For this review, take the finished solid that the model builds, in its own axes (mm). A direction names the side the tool comes from. Coordinates: 2 decimals unless noted, no trailing zeros. Loops run counter-clockwise (first coordinate to the right, second up) from the corner with the lowest first, then second, coordinate; pieces in that order, holes last. Notation, with made-up numbers: M -20,1 L 34,1 A9 cw 34,5 Z; hole C -37,13.25 d8. An arc over 180 degrees is marked long. Answer as a JSON object with one key per item and string values. Group by question number.
Item 1: Mouldability with a two-part tool opening along X and no side actions: class faces 3 (the face through (50, 4, 0)), 4 (the face through (107.95, 38, 25)), 5 (the face through (53, 5.08, 23)) as +X half, -X half, draft (parallel to the pull), parting line (faces both ways), or undercut.
Item 2: Tool access review of faces 1 (the face through (53, 38, 45.72)), 2 (the face through (53, 76.2, 25)): name each direction out of +Z, -Z, +X, -X, +Y, -Y from which nothing blocks a thin tool from reaching the whole face with its end or side.
Item 3: Add section C-C (y = 24). State the section outline as (x, z) points.
Item 4: Add section B-B (x = 29). State the section outline as (y, z) points.
Item 5: Insertion check: pin 1 (23 mm diameter, centred on y = 40.5, z = 16.5, fed in from -X); pin 2 (4 mm diameter, centred on x = 39.5, y = 38.5, fed in from -Z). Each pin has a flat end and moves straight along its axis. Give the tip position at first contact, or say it passes through.
Item 6: Add section A-A (z = 26.5). State the section outline as (x, y) points, then the cut area to 3 significant figures.
Item 7: Wall thickness on L1, parallel to Y at x = 28, z = 16; L2, parallel to X at y = 55.5, z = 29; L3, parallel to Z at x = 57, y = 38: over which ranges is each line inside the solid? List them lowest first. Write a range as from..to.
from build123d import *

# Parameters (mm, degrees)
F0_W     = 107.95
F0_H     = 76.2
F0_W_2   = 97.79
F0_H_2   = 66.04
F1_DEPTH = 50.8
F2_W     = 97.79
F2_H     = 66.04
F3_DEPTH = 45.72


with BuildPart() as f1:
    # F0 (on Top) → F1 (new body)
    with BuildSketch(Plane.XY):
        with Locations((53.975, 38.1)):
            Rectangle(F0_W, F0_H)
        with Locations((53.975, 38.1)):
            Rectangle(F0_W_2, F0_H_2, mode=Mode.SUBTRACT)
        with Locations((53.975, 38.1)):
            Rectangle(F0_W_2, F0_H_2)
    extrude(amount=F1_DEPTH)

    # F2 (on face) → F3 (cut)
    with BuildSketch(Plane(origin=(0, 0, 0), x_dir=(1, 0, 0), z_dir=(0, 0, -1))):
        with Locations((53.975, -38.1)):
            Rectangle(F2_W, F2_H)
    extrude(amount=-F3_DEPTH, mode=Mode.SUBTRACT)


solid = f1.part
From the geometry:
{
 "1": {"face 3": "draft", "face 4": "+X half", "face 5": "undercut"},
 "2": {"face 1": "-Z", "face 2": "+Z, -Z, +X, -X, +Y"},
 "3": {"outline": "M 0,0 L 5.08,0 L 5.08,45.72 L 102.87,45.72 L 102.87,0 L 107.95,0 L 107.95,50.8 L 0,50.8 Z"},
 "4": {"outline": "M 0,0 L 5.08,0 L 5.08,45.72 L 71.12,45.72 L 71.12,0 L 76.2,0 L 76.2,50.8 L 0,50.8 Z"},
 "5": {"pin 1": "stops at x = 0", "pin 2": "stops at z = 45.72"},
 "6": {"outline": "M 0,0 L 107.95,0 L 107.95,76.2 L 0,76.2 Z; hole M 5.08,5.08 L 102.87,5.08 L 102.87,71.12 L 5.08,71.12 Z", "area": "1,770 mm²"},
 "7": {"L1": "y = 0..5.08, 71.12..76.2", "L2": "x = 0..5.08, 102.87..107.95", "L3": "z = 45.72..50.8"}
}
